```python
from build123d import *

# Parameters (mm, degrees)
F1_DEPTH = 63.5
F2_DEPTH = 25.4
F3_DEPTH = 7.9375
F0_W     = 3.175
F0_H     = 19.05
F0_W_2   = 25.3145909364
F5_DEPTH = 25.4
F7_R     = 6.35


with BuildPart() as f1:
    # F0 (on Front) → F1 (new body, symmetric)
    with BuildSketch(Plane.XZ):
        Polygon((-41.275, -9.525), (41.275, -9.525), (41.275, 9.525), (22.225, 9.525), (-41.275, 9.525), align=None)
    extrude(amount=F1_DEPTH, both=True)

    # F0 (on Front) → F2 (join, symmetric)
    with BuildSketch(Plane.XZ):
        with BuildLine():
            Line((22.225, 9.525), (41.275, 9.525))
            Line((41.275, 9.525), (41.275, 27.0002))
            ThreePointArc((41.275, 27.0002), (45.9246798487, 38.2255201513), (57.15, 42.8752))
            Line((57.15, 42.8752), (57.15, 61.9252))
            add(Edge.make_bspline(
                [(52.766737565, 61.6490475339), (54.2109947937, 61.7540958796), (55.6720672383, 61.8462382858), (57.15, 61.9252)],
                knots=[108.6209629864, 108.6209629864, 108.6209629864, 108.6209629864, 111.5045361635, 111.5045361635, 111.5045361635, 111.5045361635], degree=3))
            ThreePointArc((52.766737565, 61.6490475339), (30.9503715146, 50.0942488488), (22.225, 27.0002))
            Line((22.225, 27.0002), (22.225, 9.525))
        make_face()
    extrude(amount=F2_DEPTH, both=True)

    # F0 (on Front) → F3 (join, symmetric)
    with BuildSketch(Plane.XZ):
        with BuildLine():
            add(Edge.make_bspline(
                [(-41.275, 9.525), (-32.1805033195, 35.4221321522), (-1.6368101652, 57.6919943344), (52.766737565, 61.6490475339)],
                knots=[0, 0, 0, 0, 108.6209629864, 108.6209629864, 108.6209629864, 108.6209629864], degree=3))
            Line((-41.275, 9.525), (22.225, 9.525))
            Line((22.225, 9.525), (22.225, 27.0002))
            ThreePointArc((22.225, 27.0002), (30.9503715146, 50.0942488488), (52.766737565, 61.6490475339))
        make_face()
    extrude(amount=F3_DEPTH, both=True)



with BuildPart() as f4:
    # F0 (on Front) → F4 (revolve)
    with BuildSketch(Plane.XZ):
        Polygon((85.6395909364, 66.675), (85.725, 38.354), (111.125, 38.354), (111.125, 66.675), align=None)
    revolve(axis=Axis((85.6822954682, 0, 52.5145), (0.0030157366, 0, -0.9999954527)))


with BuildPart() as f1_1:
    add(f1.part)

    add(f4.part)  # F5 merges F4
    # F0 (on Front) → F5 (join, symmetric)
    with BuildSketch(Plane.XZ):
        with Locations((58.7375, 52.4002)):
            Rectangle(F0_W, F0_H)
        with Locations((72.9822954682, 52.4002)):
            Rectangle(F0_W_2, F0_H)
    extrude(amount=F5_DEPTH, both=True)

    # F0 (on Front) → F6 (revolve)
    with BuildSketch(Plane.XZ):
        Polygon((85.6395909364, 66.675), (85.725, 38.354), (111.125, 38.354), (111.125, 66.675), align=None)
    revolve(axis=Axis((85.6822954682, 0, 52.5145), (0.0030157366, 0, -0.9999954527)))

    # F7
    f7_edges = [f1_1.edges().sort_by_distance(p)[0] for p in [
        (-41.275, -63.5, 0),
        (41.275, -63.5, 0),
        (41.275, 63.5, 0),
        (-41.275, 63.5, 0),
    ]]
    fillet(f7_edges, radius=F7_R)


solid = f1_1.part
```
Source: CAD feature listing. Evaluate the final solid. Frame: model axes, mm. A direction names the side the tool comes from. Coordinates: 2 decimals unless noted, no trailing zeros. Loops run counter-clockwise (first coordinate to the right, second up) from the corner with the lowest first, then second, coordinate; pieces in that order, holes last. Notation, with made-up numbers: (-11.75, 31) -> (26.25, 31) arc R22 cw to (26.25, 55) -> close; hole circle Ø1 at (15.5, 88.5). An arc over 180 degrees is marked (long way). One line per item, written item: value. Start each with the question number.
Q1. Section query A-A, the plane z = 0. Return the cut outline in (x, y) (3 decimals).
Q2. Section query B-B, the plane y = -46. Return the cut outline in (x, z) (3 decimals), and give its area (3 significant figures).
Q3. Line query: line 1 along X through (y, z) = (-46, 3) (3 decimals); line 2 along Z through (x, y) = (20.5, -56) (3 decimals); line 3 along Y through (x, z) = (38, 38.5). Output: solid intervals per line, ascending.
Q4. Mould query, pull axis X, two halves, no side actions, for faces 1 (the face through (-1, -1, -9.525)), 2 (the face through (45.8, -0.4, 38.1)), 3 (the face through (31.185, -16.791, 50.358)). Classes: pulls with the +X half, pulls with the -X half, needs draft (parallel to the pull), parting line crosses it, or undercut.
Q5. Set-up query: faces 4 (the face through (109.95, -7.64, 52.71)), 5 (the face through (60, 2, 42.875)), 6 (the face through (22.225, -17, 18)). Return all of +Z, -Z, +X, -X, +Y, -Y with unobstructed straight access to the full face (end or side cutting, diameter ignored); none if empty.
Q6. Contact query for flat-ended pins moving along their axis: P1, Ø6, axis at y = -17, z = 42, coming from the +X side; P2, Ø8, axis at x = 44, y = -41.5, coming from the +Z side (3 decimals); P3, Ø14, axis at x = 72, y = 12.5, coming from the -Z side. Output: stop coordinate, or through.
Results:
1. outline: (-41.275, -57.15) arc R6.35 ccw to (-34.925, -63.5) -> (34.925, -63.5) arc R6.35 ccw to (41.275, -57.15) -> (41.275, 57.15) arc R6.35 ccw to (34.925, 63.5) -> (-34.925, 63.5) arc R6.35 ccw to (-41.275, 57.15) -> close
2. outline: (-41.275, -9.525) -> (41.275, -9.525) -> (41.275, 9.525) -> (-41.275, 9.525) -> close
2. area: 1,570 mm^2
3. line 1: -41.275 to 41.275
3. line 2: -9.525 to 9.525
3. line 3: -25.4 to 25.4
4. face 1: needs draft
4. face 2: undercut
4. face 3: pulls with the -X half
5. face 4: none
5. face 5: -Z
5. face 6: +Z, -X, -Y
6. P1: x = 106.92
6. P2: z = 9.525
6. P3: z = 38.22
